Read the model definition and answer for the solid it produces. Units are mm, in the model's axes. A direction names the side the tool comes from. Round coordinates to 2 decimals unless told otherwise and drop trailing zeros. Order: outer loops, then holes, each group sorted by start corner. A loop starts at its lowest first (then second) coordinate and runs counter-clockwise, first axis right, second up. Notation, with made-up numbers: (67.5, 89.5) -> (104.5, 89.5) arc R9 ccw to (104.5, 98.5) -> close; hole circle Ø11 at (13, 0.5). An arc over 180 degrees is marked (long way). Answer as a JSON object with one key per item and string values. Group by question number.
Item 1: Consider probe 1 along Y at (x, z) = (-16, 26); probe 2 along Z at (x, y) = (-6, -9.25); probe 3 along Z at (x, y) = (-18.5, -9.5). Determine where each line is inside the solid, lowest interval first. Write a range as from..to.
Item 2: Section B-B, the plane x = -4.5 is taken. Write down the section's boundary in (y, z) (1 decimal).
Item 3: For faces 5 (the flat face through (-30, -7, 0)), 6 (the flat face through (-14.79, -9.573, -3.949)), 7 (the flat face through (-15, -7.9, 4)), 8 (the flat face through (-15, -7, 24.865)), determine the directions among +Z, -Z, +X, -X, +Y, -Y from which every point of the face is accessible in a straight line to the end or side of a thin tool.
Item 4: Section D-D, the plane z = 10 is taken. Write down the section's boundary in (x, y), plus the area to 3 significant figures.
Item 5: The mould has two halves that part along Y. Classify faces 1 (the flat face through (-15, -7.855, 16)), 2 (the cylindrical face through (-0.9, -12.91, -8.43)), 3 (the flat face through (-15, -4.3, 0)), 4 (the flat face through (-26, -15.371, 22)): pulls with the +Y half, pulls with the -Y half, needs draft (parallel to the pull), parting line crosses it, or undercut.
Item 6: Given P1, Ø5, axis at x = -18.5, z = 18.5, coming from the +Y side; P2, Ø0.5, axis at x = -20, y = -7, coming from the -Z side; P3, Ø1.2, axis at x = -20, y = -7, coming from the +Z side (3 decimals), each flat-ended and moving along its own axis, determine where each tip first touches the part or whether it passes through.
Item 7: Section A-A, the plane y = -13.75 is taken. Write down the section's boundary in (x, z), plus the area to 3 significant figures.
Item 8: Section C-C, the plane y = -5.25 is taken. Write down the section's boundary in (x, z), plus the area to 3 significant figures.
Autodesk Inventor part; units mm, degrees
ref_plane "YZ Plane" through (0, 0, 0) normal (1, 0, 0) x (0, 1, 0)
ref_plane "XZ Plane" through (0, 0, 0) normal (0, 1, 0) x (-1, 0, 0)
ref_plane "XY Plane" through (0, 0, 0) normal (0, 0, 1) x (1, 0, 0)
sketch "Sketch1" plane through (0, 0, 0) normal (1, 0, 0) x (0, 1, 0)
  line L0 (-10.3707, -4.7464) -> (-8.7536, -3.1293)
  line L1 (-10.3707, 15.395) -> (-8.7381, 17.0275)
  arc A0 (-7.8549, 16.6) -> (-8.7381, 17.0275) centre (-8.4, 16.6) ccw
  line L2 (-7.8549, 16.6) -> (-7.8549, 15.135)
  line L3 (-7.8549, 15.135) -> (-6.3429, 15.135)
  line L4 (-6.3429, 15.135) -> (-4.3451, 17.1329)
  line L5 (-4.3451, 17.1329) -> (-4.3451, 22.8671)
  line L6 (-4.3451, 22.8671) -> (-6.3429, 24.865)
  line L7 (-6.3429, 24.865) -> (-7.8549, 24.865)
  line L8 (-7.8549, 24.865) -> (-7.8549, 23.8568)
  arc A1 (-9.0499, 23.3618) -> (-7.8549, 23.8568) centre (-8.5549, 23.8568) ccw
  line L9 (-9.0499, 23.3618) -> (-10.3707, 24.6827)
  line L10 (-10.3707, 24.6827) -> (-10.3707, 30.0707)
  line L11 (-10.3707, 30.0707) -> (-11.3707, 30.0707)
  line L12 (-11.9747, -9.2902) -> (-10.3707, -9.2902)
  arc A2 (-7.9, -3.4828) -> (-8.7536, -3.1293) centre (-8.4, -3.4828) ccw
  line L13 (-7.9, -3.4828) -> (-7.9, -4.9101)
  line L14 (-7.9, -4.9101) -> (-6.3243, -4.9101)
  line L15 (-6.3243, -4.9101) -> (-4.3, -2.8858)
  line L16 (-4.3, -2.8858) -> (-4.3, 2.8858)
  line L17 (-4.3, 2.8858) -> (-6.3243, 4.9101)
  line L18 (-6.3243, 4.9101) -> (-7.9, 4.9101)
  line L19 (-7.9, 4.9101) -> (-7.9, 3.4828)
  arc A3 (-8.7536, 3.1293) -> (-7.9, 3.4828) centre (-8.4, 3.4828) ccw
  line L20 (-8.7536, 3.1293) -> (-10.3707, 4.7464)
  line L21 (-10.3707, 15.395) -> (-10.3707, 4.7464)
  line L22 (-10.3707, 30.0707) -> (-15.3707, 30.0707)
  line L23 (-15.3707, 30.0707) -> (-15.3707, -9.2902)
  line L24 (-15.3707, -9.2902) -> (-10.3707, -9.2902)
  line L25 (-10.3707, 24.6827) -> (-10.3707, 30.0707)
  line L26 (-10.3707, -9.2902) -> (-10.3707, -4.7464)
  line L27 (-10.3707, 4.7464) -> (-10.3707, 15.395)
  point P0 (0, 0)
  point P1 (-7.8549, 16.6)
  point P2 (-9.0499, 23.3618)
  dimension "d0" = 5
extrude "Extrusion1" add sketch "Sketch1" against normal blind 30
sketch "Sketch2" plane through (0, -15.3707, -9.2902) normal (0, -1, 0) x (1, 0, 0)
  line L0 (-30, 0) -> (-30, 39.3609)
  circle A0 centre (-30, 39.3609) radius 22.5
  circle A1 centre (-40.6066, 49.9675) radius 4
  point P0 (0, 9.2902)
  dimension "d3" = 45
  dimension "d4" = 8
  dimension "d5" = 10.6066
  dimension "d6" = 10.6066
extrude "Extrusion2" add sketch "Sketch2" against normal blind 5
fillet "Fillet1" radius 30 1 edges at (-7.5, -12.8707, 30.0707)
fillet "Fillet2" radius 3 1 edges at (0, -12.8707, 30.0707)
sketch "Sketch3" plane through (-30, 0, 0) normal (-1, 0, 0) x (0, 0, 1)
  line L0 (7.5707, -15.3707) -> (7.5707, -10.3707)
  line L1 (-9.2902, -10.3707) -> (-9.2902, -15.3707)
  line L2 (7.5707, -15.3707) -> (-9.2902, -15.3707)
  line L3 (-9.2902, -15.3707) -> (-9.2902, -10.3707)
  line L4 (-9.2902, -10.3707) -> (7.5707, -10.3707)
  line L5 (7.5707, -10.3707) -> (7.5707, -15.3707)
  point P0 (0, 0)
extrude "Extrusion3" cut sketch "Sketch3" against normal blind 0.75
fillet "Fillet3" radius 30 1 edges at (-29.25, -12.8707, 7.5707)
fillet "Fillet4" radius 3 1 edges at (0, -12.8707, -9.2902)
fillet "Fillet5" radius 3 1 edges at (-29.25, -12.8707, -9.2902)
equation "\"d6\" = d5"
properties part number "Webcam Mount"
Values found:
{
 "1": {"probe 1": "-15.37..-10.37", "probe 2": "-3.63..3.63, 16.52..23.56", "probe 3": "-3.88..3.88, 16.27..23.81"},
 "2": {"outline": "(-15.4, -9.3) -> (-10.4, -9.3) -> (-10.4, -4.7) -> (-8.8, -3.1) arc R0.5 cw to (-7.9, -3.5) -> (-7.9, -4.9) -> (-6.3, -4.9) -> (-4.3, -2.9) -> (-4.3, 2.9) -> (-6.3, 4.9) -> (-7.9, 4.9) -> (-7.9, 3.5) arc R0.5 cw to (-8.8, 3.1) -> (-10.4, 4.7) -> (-10.4, 15.4) -> (-8.7, 17) arc R0.5 cw to (-7.9, 16.6) -> (-7.9, 15.1) -> (-6.3, 15.1) -> (-4.3, 17.1) -> (-4.3, 22.9) -> (-6.3, 24.9) -> (-7.9, 24.9) -> (-7.9, 23.9) arc R0.7 cw to (-9, 23.4) -> (-10.4, 24.7) -> (-10.4, 33.5) -> (-15.4, 33.5) -> close"},
 "3": {"face 5": "+Z, -Z, -X, +Y", "face 6": "-Z, +X, -X", "face 7": "+X, -X", "face 8": "+Z, +X, -X, +Y"},
 "4": {"outline": "(-40.59, -15.37) -> (0, -15.37) -> (0, -10.37) -> (-40.59, -10.37) -> close", "area": "203 mm2"},
 "5": {"face 1": "undercut", "face 2": "needs draft", "face 3": "pulls with the +Y half", "face 4": "pulls with the -Y half"},
 "6": {"P1": "y = -4.35", "P2": "z = -4.91", "P3": "z = 24.865"},
 "7": {"outline": "(-42.39, 11.29) arc R30 cw to (-29.69, -6.97) arc R3 ccw to (-26.77, -9.29) -> (-3, -9.29) arc R3 ccw to (0, -6.29) -> (0, 28.46) arc R3 ccw to (-1.28, 30.92) arc R30 cw to (-10.31, 40.96) arc R22.5 ccw (long way) to start; hole circle Ø8 at (-40.61, 40.68)", "area": "2,390 mm2"},
 "8": {"outline": "(-30, -3.84) -> (0, -3.84) -> (0, 3.84) -> (-30, 3.84) -> close; (-30, 16.23) -> (0, 16.23) -> (0, 23.77) -> (-30, 23.77) -> close", "area": "456 mm2"}
}
